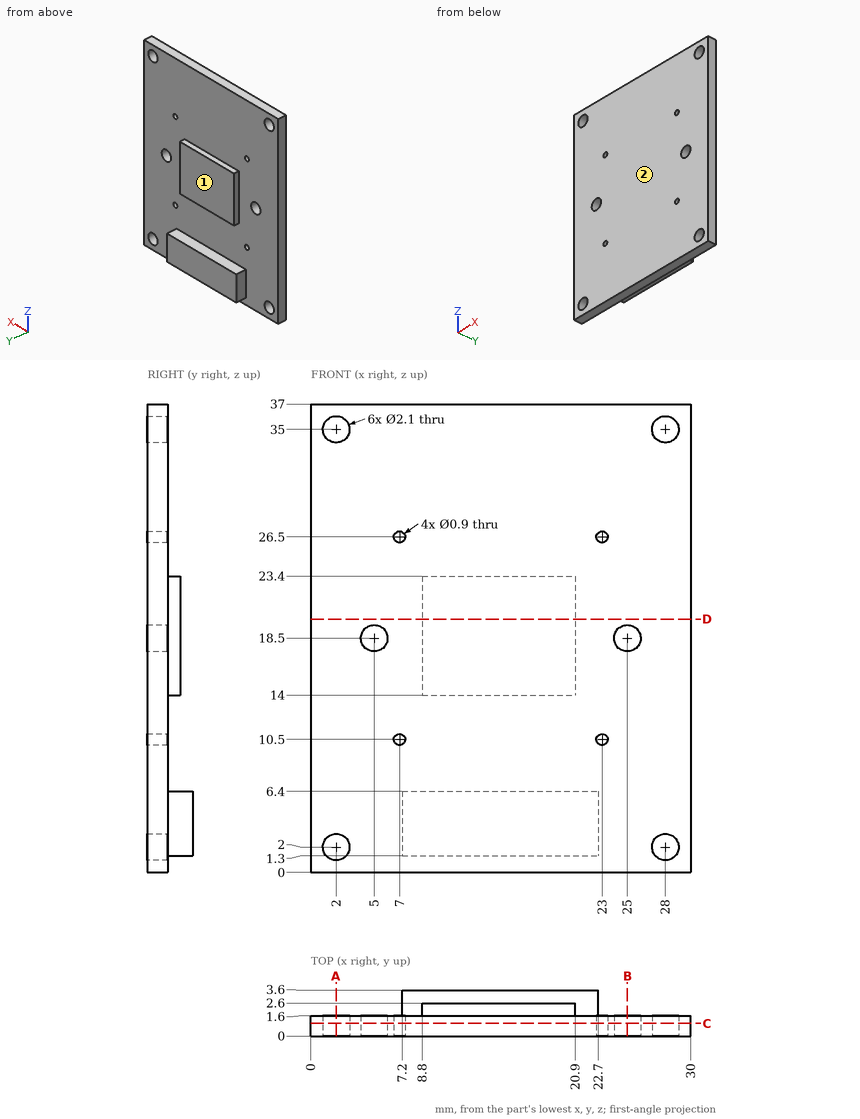
Geometry check sheet. Reference: drawing and pictorial views, mm from the part's lowest x, y, z. A direction names the side the tool comes from. Coordinates: 2 decimals unless noted, no trailing zeros. Order: outer loops, then holes, each group sorted by start corner. A loop starts at its lowest first (then second) coordinate and runs counter-clockwise, first axis right, second up.
Item 1: Section check A-A, the plane x = 2. Enter the section's corners in (y, z).
Filled in:
outline: (0, 0) - (1.6, 0) - (1.6, 0.95) - (0, 0.95) - close; (0, 3.05) - (1.6, 3.05) - (1.6, 33.95) - (0, 33.95) - close; (0, 36.05) - (1.6, 36.05) - (1.6, 37) - (0, 37) - close
Item 2: Section check B-B, the plane x = 25. Enter the section's corners in (y, z), then the cut area to 3 significant figures.
Filled in:
outline: (0, 0) - (1.6, 0) - (1.6, 17.45) - (0, 17.45) - close; (0, 19.55) - (1.6, 19.55) - (1.6, 37) - (0, 37) - close
area: 55.8 mm2
Item 3: Material ranges on L1, parallel to X at y = 1.1, z = 26.5; L2, parallel to X at y = 0.9, z = 2; L3, parallel to Z at x = 11.5, y = 3.05, recorded low to high.
Filled in:
L1: x = 0 to 6.55, 7.45 to 22.55, 23.45 to 30
L2: x = 0 to 0.95, 3.05 to 26.95, 29.05 to 30
L3: z = 1.3 to 6.4
Item 4: Section check D-D, the plane z = 20. Enter the section's corners in (x, y).
Filled in:
outline: (0, 0) - (30, 0) - (30, 1.6) - (20.9, 1.6) - (20.9, 2.6) - (8.8, 2.6) - (8.8, 1.6) - (0, 1.6) - close
Item 5: Access from +Z, -Z, +X, -X, +Y, -Y to the whole of each face (thin tool, end or side, straight path). Record for the marked faces 1 and 2.
Filled in:
face 1: +Z, +X, -X, +Y
face 2: +Z, -Z, +X, -X, -Y
Item 6: Depth check by flat-ended pin: pin 1 (2.5 mm diameter, centred on x = 2, z = 35, fed in from -Y); pin 2 (0.5 mm diameter, centred on y = 2, z = 18, fed in from +X); pin 3 (2.5 mm diameter, centred on x = 28, z = 2, fed in from +Y); pin 4 (3 mm diameter, centred on x = 14.5, z = 17, fed in from +Y). Enter the tip coordinate at first touch or a pass-through.
Filled in:
pin 1: stops at y = 0
pin 2: stops at x = 20.9
pin 3: stops at y = 1.6
pin 4: stops at y = 2.6
Item 7: Section check C-C, the plane y = 1. Give the number of separate pieces and of enclosed holes in the cut face, then the cut area to 3 significant figures.
Filled in:
separate pieces: 1
enclosed holes: 10
area: 1,090 mm2
